from build123d import *

# Parameters (mm, degrees)
SKETCH1_R           = 8.5
SKETCH1_R_2         = 4
BOSS_EXTRUDE1_DEPTH = 7
SKETCH3_R           = 25
SKETCH3_R_2         = 4
BOSS_EXTRUDE3_DEPTH = 6
SKETCH4_R           = 8.5
SKETCH4_R_2         = 4
BOSS_EXTRUDE4_DEPTH = 7
SKETCH5_R           = 8.5
SKETCH5_R_2         = 4
BOSS_EXTRUDE5_DEPTH = 7
BOSS_EXTRUDE6_START = -3
SKETCH6_R           = 8.5
BOSS_EXTRUDE6_DEPTH = 3


with BuildPart() as part:
    # Sketch1 → Boss-Extrude1 (new body)
    with BuildSketch(Plane(origin=(0, 0, 0), x_dir=(1, 0, 0), z_dir=(0, 1, 0))):
        with Locations(Location((0, 0, 0), (0, 0, 270))):
            Circle(SKETCH1_R)
        with Locations(Location((0, 0, 0), (0, 0, 270))):
            Circle(SKETCH1_R_2, mode=Mode.SUBTRACT)
    extrude(amount=BOSS_EXTRUDE1_DEPTH)

    # Sketch3 → Boss-Extrude3 (add)
    with BuildSketch(Plane(origin=(0, 7, 0), x_dir=(1, 0, 0), z_dir=(0, 1, 0))):
        with Locations(Location((0, 0, 0), (0, 0, 270))):
            Circle(SKETCH3_R)
        with Locations(Location((0, 0, 0), (0, 0, 270))):
            Circle(SKETCH3_R_2, mode=Mode.SUBTRACT)
    extrude(amount=BOSS_EXTRUDE3_DEPTH)

    # Sketch4 → Boss-Extrude4 (add)
    with BuildSketch(Plane(origin=(0, 13, 0), x_dir=(1, 0, 0), z_dir=(0, 1, 0))):
        with Locations(Location((0, -1, 0), (0, 0, 270))):
            Circle(SKETCH4_R)
        with Locations(Location((0, 0, 0), (0, 0, 270))):
            Circle(SKETCH4_R_2, mode=Mode.SUBTRACT)
    extrude(amount=BOSS_EXTRUDE4_DEPTH)

    # Sketch5 → Boss-Extrude5 (add)
    with BuildSketch(Plane(origin=(0, 20, 0), x_dir=(1, 0, 0), z_dir=(0, 1, 0))):
        with Locations(Location((0, 1, 0), (0, 0, 186.756327031))):
            Circle(SKETCH5_R)
        with Locations(Location((0, 0, 0), (0, 0, 270))):
            Circle(SKETCH5_R_2, mode=Mode.SUBTRACT)
    extrude(amount=BOSS_EXTRUDE5_DEPTH)

    # Sketch6 → Boss-Extrude6 (add)
    with BuildSketch(Plane(origin=(0, 27, 0), x_dir=(1, 0, 0), z_dir=(0, 1, 0)).offset(BOSS_EXTRUDE6_START)):
        with Locations(Location((0, 1, 0), (0, 0, 186.756327031))):
            Circle(SKETCH6_R)
    extrude(amount=BOSS_EXTRUDE6_DEPTH)


solid = part.part
The model under review builds one solid part; all positions refer to its coordinate system, in mm. A direction names the side the tool comes from. Give positions to 0.01 mm unless a question says otherwise; leave off trailing zeros. Loops run counter-clockwise (first coordinate to the right, second up) from the corner with the lowest first, then second, coordinate; pieces in that order, holes last. Notation, with made-up numbers: (-15, 29) -> (41, 29) arc R26 ccw to (41, 49) -> close; hole circle Ø6 at (18.5, -36.5). An arc over 180 degrees is marked (long way). Answer as a JSON object with one key per item and string values. Group by question number.
Q1. Wall thickness on line 1 along X through (y, z) = (8.25, 0); line 2 along Y through (x, z) = (-1.5, -7.5); line 3 along Z through (x, y) = (0, 18.5): over which ranges is each line inside the solid? List them lowest first.
Q2. Tool access review of faces 4 (the flat face through (1, 20, 8)), 5 (the cylindrical face through (8.428, 16.451, -0.107)), 6 (the flat face through (0, 20, -8)): name each direction out of +Z, -Z, +X, -X, +Y, -Y from which nothing blocks a thin tool from reaching the whole face with its end or side.
Q3. Take a section at C-C (y = 15). Write out the cut boundary in (x, z), plus the area to 3 significant figures.
Q4. Take a section at B-B (z = 1). Write out the cut boundary in (x, y).
Q5. Insertion check: pin 1 (3 mm diameter, centred on y = 9, z = -12, fed in from +X); pin 2 (1.5 mm diameter, centred on x = -2.5, z = 16, fed in from +Y); pin 3 (2.5 mm diameter, centred on x = 1, z = 1, fed in from -Y). Each pin has a flat end and moves straight along its axis. Give the tip position at first contact, or say it passes through.
Q6. Draft analysis for pull direction Z (two halves, no side actions). For faces 1 (the flat face through (0, 24, 0)), 2 (the flat face through (0, 27, -1)), 3 (the cylindrical face through (6.897, 23.451, 3.968)), state which applies: pulls with the +Z half, pulls with the -Z half, needs draft (parallel to the pull), parting line crosses it, or undercut.
Q7. Take a section at A-A (y = 8.5). Write out the cut boundary in (x, z).
Q8. Take a section at D-D (x = 9.5). Write out the cut boundary in (y, z), plus the area to 3 significant figures.
Answer below:
{
 "1": {"line 1": "x = -25 to -4, 4 to 25", "line 2": "y = 0 to 13, 20 to 27", "line 3": "z = -7.5 to -4, 4 to 9.5"},
 "2": {"face 4": "+Z, +Y", "face 5": "none", "face 6": "-Z"},
 "3": {"outline": "circle Ø17 at (0, 1); hole circle Ø8 at (0, 0)", "area": "177 mm2"},
 "4": {"outline": "(-24.98, 7) -> (-8.44, 7) -> (-8.44, 0) -> (-3.87, 0) -> (-3.87, 24) -> (3.87, 24) -> (3.87, 0) -> (8.44, 0) -> (8.44, 7) -> (24.98, 7) -> (24.98, 13) -> (8.5, 13) -> (8.5, 20) -> (8.26, 20) -> (8.26, 27) -> (-8.26, 27) -> (-8.26, 20) -> (-8.5, 20) -> (-8.5, 13) -> (-24.98, 13) -> close"},
 "5": {"pin 1": "stops at x = 22.69", "pin 2": "stops at y = 13", "pin 3": "stops at y = 24"},
 "6": {"face 1": "undercut", "face 2": "needs draft", "face 3": "parting line crosses it"},
 "7": {"outline": "circle Ø50 at (0, 0); hole circle Ø8 at (0, 0)"},
 "8": {"outline": "(7, -23.12) -> (13, -23.12) -> (13, 23.12) -> (7, 23.12) -> close", "area": "277 mm2"}
}
